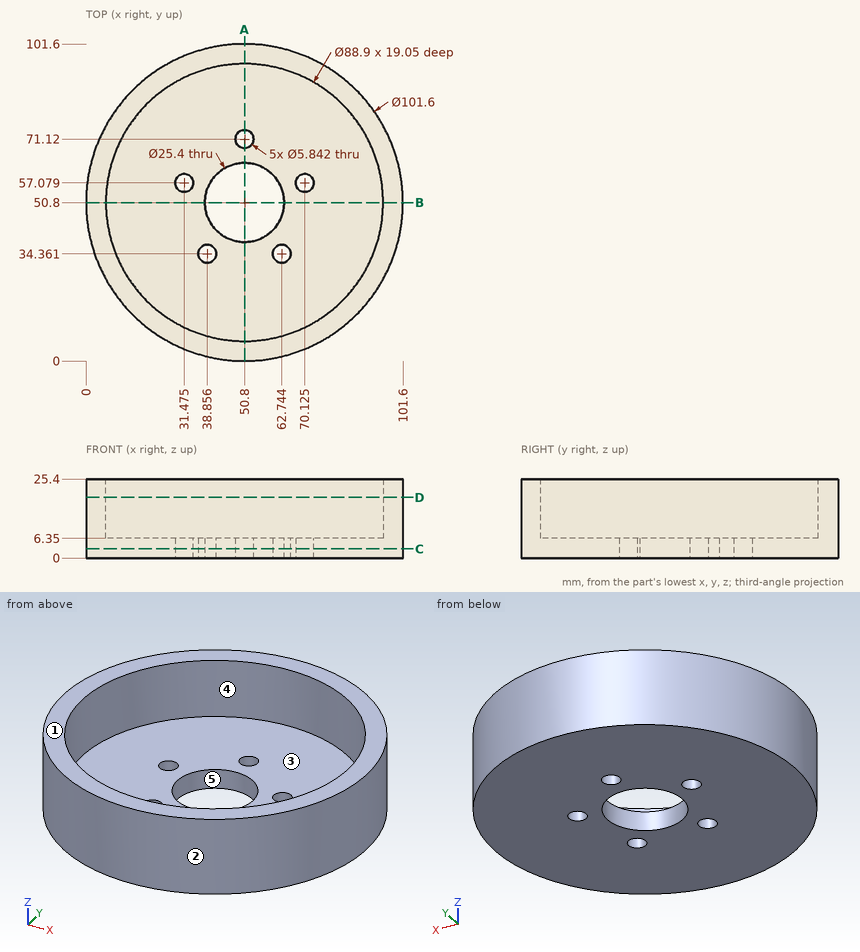
Answer from the drawing. Dimensions are ordinates in mm from the lowest x, y and z of the part. A direction names the side the tool comes from. Coordinates: 2 decimals unless noted, no trailing zeros. Write each loop counter-clockwise with the first axis right and the second up, starting at its lowest first coordinate (ties: lowest second). Pieces come first, ordered by that corner, then holes. Notation, with made-up numbers: (83.5, 11.5) - (92.5, 11.5) arc R30 cw to (92.5, 34.5) - close; hole circle Ø9 at (-3, -23.5). An arc over 180 degrees is marked (long way). One line per question, with ' | ' between items.
Q1. For the marked faces 4 and 5, determine the directions among +Z, -Z, +X, -X, +Y, -Y from which every point of the face is accessible in a straight line to the end or side of a thin tool.
Result set:
face 4: +Z | face 5: +Z, -Z
Q2. Find section D-D, the plane z = 19.5. Write down the section's boundary in (x, y), plus the area to 3 significant figures.
Result set:
outline: circle Ø101.6 at (50.8, 50.8); hole circle Ø88.9 at (50.8, 50.8) | area: 1,900 mm^2
Q3. Find section A-A, the plane x = 50.8. Write down the section's boundary in (y, z).
Result set:
outline: (0, 0) - (38.1, 0) - (38.1, 6.35) - (6.35, 6.35) - (6.35, 25.4) - (0, 25.4) - close; (63.5, 0) - (68.2, 0) - (68.2, 6.35) - (63.5, 6.35) - close; (74.04, 0) - (101.6, 0) - (101.6, 25.4) - (95.25, 25.4) - (95.25, 6.35) - (74.04, 6.35) - close
Q4. Consider L1, parallel to Y at x = 50.8, z = 1.5; L2, parallel to X at y = 54, z = 13 (1 decimal); L3, parallel to Z at x = 68.5, y = 21.5. Determine where each line is inside the solid, lowest interval first. Write a range as [from, to].
Result set:
L1: [0, 38.1], [63.5, 68.2], [74.04, 101.6] | L2: [0.1, 6.5], [95.1, 101.5] | L3: [0, 6.35]
Q5. Find section C-C, the plane z = 3. Write down the section's boundary in (x, y) (1 decimal), plus the area to 3 significant figures.
Result set:
outline: circle Ø101.6 at (50.8, 50.8); hole circle Ø5.8 at (31.5, 57.1); hole circle Ø5.8 at (38.9, 34.4); hole circle Ø25.4 at (50.8, 50.8); hole circle Ø5.8 at (50.8, 71.1); hole circle Ø5.8 at (62.7, 34.4); hole circle Ø5.8 at (70.1, 57.1) | area: 7,470 mm^2
Q6. Determine the mould class of the marked faces 1, 2 and 3 for opening direction Y: +Y half, -Y half, draft (parallel to the pull), parting line (faces both ways), or undercut.
Result set:
face 1: draft | face 2: parting line | face 3: undercut
Q7. Each of these flat-tipped pins is pushed along its axis until it touches: P1, Ø6, axis at x = 37, z = 4, coming from the -Y side; P2, Ø6, axis at x = 43, y = 90, coming from the +Z side; P3, Ø10, axis at x = 62.5, z = 7, coming from the -Y side; P4, Ø23, axis at x = 50.8, y = 50.8, coming from the +Z side. Where does it stop, or does it pass through?
Result set:
P1: y = 1.16 | P2: z = 6.35 | P3: y = 0.44 | P4: through
Q8. Find section B-B, the plane y = 50.8. Write down the section's boundary in (x, z), plus the area to 3 significant figures.
Result set:
outline: (0, 0) - (38.1, 0) - (38.1, 6.35) - (6.35, 6.35) - (6.35, 25.4) - (0, 25.4) - close; (63.5, 0) - (101.6, 0) - (101.6, 25.4) - (95.25, 25.4) - (95.25, 6.35) - (63.5, 6.35) - close | area: 726 mm^2
